```python
from build123d import *

# Parameters (mm, degrees)
V4_UPPER_DECK_221X142_PROFILE_W  = 221
V4_UPPER_DECK_221X142_PROFILE_H  = 142
V4_UPPER_DECK_5MM_DEPTH          = 5
V4_FIVE_SUPPORT_POSTS_PROFILE_W  = 16
V4_FIVE_SUPPORT_POSTS_PROFILE_H  = 16
V4_FIVE_SUPPORT_POSTS_59MM_DEPTH = 59
V4_UPPER_TWO_CABLE_SLOTS_DEPTH   = 5.5
V4_FIVE_M3_PILOTS_PROFILE_R      = 1.4
V4_POST_PILOT_HOLES_DEPTH        = 14


with BuildPart() as part:
    # V4_upper_deck_221x142_profile → V4_upper_deck_5mm (new body)
    with BuildSketch(Plane(origin=(0, 4, 0), x_dir=(1, 0, 0), z_dir=(0, 1, 0))):
        with Locations((12.5, -115)):
            Rectangle(V4_UPPER_DECK_221X142_PROFILE_W, V4_UPPER_DECK_221X142_PROFILE_H)
    extrude(amount=-V4_UPPER_DECK_5MM_DEPTH)

    # V4_five_support_posts_profile → V4_five_support_posts_59mm (add)
    with BuildSketch(Plane(origin=(0, -1, 0), x_dir=(1, 0, 0), z_dir=(0, 1, 0))):
        with Locations((-85, -60)):
            Rectangle(V4_FIVE_SUPPORT_POSTS_PROFILE_W, V4_FIVE_SUPPORT_POSTS_PROFILE_H)
        with Locations((110, -60)):
            Rectangle(V4_FIVE_SUPPORT_POSTS_PROFILE_W, V4_FIVE_SUPPORT_POSTS_PROFILE_H)
        with Locations((-85, -171)):
            Rectangle(V4_FIVE_SUPPORT_POSTS_PROFILE_W, V4_FIVE_SUPPORT_POSTS_PROFILE_H)
        with Locations((110, -171)):
            Rectangle(V4_FIVE_SUPPORT_POSTS_PROFILE_W, V4_FIVE_SUPPORT_POSTS_PROFILE_H)
        with Locations((12.5, -130)):
            Rectangle(V4_FIVE_SUPPORT_POSTS_PROFILE_W, V4_FIVE_SUPPORT_POSTS_PROFILE_H)
    extrude(amount=-V4_FIVE_SUPPORT_POSTS_59MM_DEPTH)

    # V4_upper_two_cable_slots_profile → V4_upper_two_cable_slots (cut)
    with BuildSketch(Plane(origin=(0, 4, 0), x_dir=(1, 0, 0), z_dir=(0, 1, 0))):
        with BuildLine():
            Line((-11, -51), (-5, -51))
            ThreePointArc((-5, -51), (-1, -55), (-5, -59))
            Line((-5, -59), (-11, -59))
            ThreePointArc((-11, -59), (-15, -55), (-11, -51))
        make_face()
        with BuildLine():
            Line((20, -51), (26, -51))
            ThreePointArc((26, -51), (30, -55), (26, -59))
            Line((26, -59), (20, -59))
            ThreePointArc((20, -59), (16, -55), (20, -51))
        make_face()
    extrude(amount=-V4_UPPER_TWO_CABLE_SLOTS_DEPTH, mode=Mode.SUBTRACT)

    # V4_five_M3_pilots_profile → V4_post_pilot_holes (cut)
    with BuildSketch(Plane(origin=(0, -60, 0), x_dir=(1, 0, 0), z_dir=(0, 1, 0))):
        with Locations(Location((-85, -60, 0), (0, 0, 270))):
            Circle(V4_FIVE_M3_PILOTS_PROFILE_R)
        with Locations(Location((110, -60, 0), (0, 0, 270))):
            Circle(V4_FIVE_M3_PILOTS_PROFILE_R)
        with Locations(Location((-85, -171, 0), (0, 0, 270))):
            Circle(V4_FIVE_M3_PILOTS_PROFILE_R)
        with Locations(Location((110, -171, 0), (0, 0, 270))):
            Circle(V4_FIVE_M3_PILOTS_PROFILE_R)
        with Locations(Location((12.5, -130, 0), (0, 0, 270))):
            Circle(V4_FIVE_M3_PILOTS_PROFILE_R)
    extrude(amount=V4_POST_PILOT_HOLES_DEPTH, mode=Mode.SUBTRACT)


solid = part.part
```
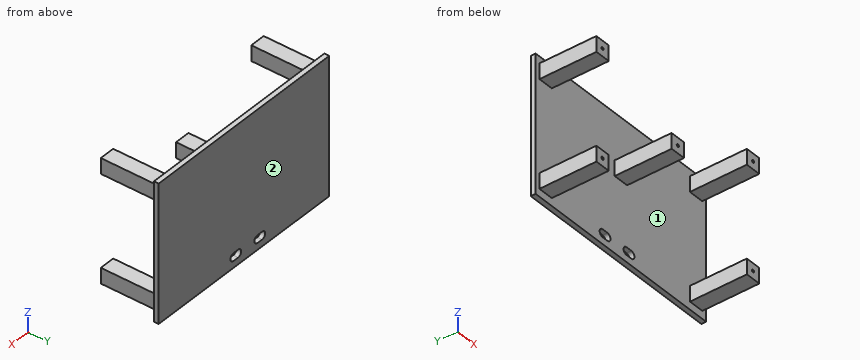
The listing builds one solid part. Answer for the finished solid, in the listing's coordinates (mm). Face numbers are marked on the shaded views. Coordinates: 2 decimals unless noted, no trailing zeros. Order: outer loops, then holes, each group sorted by start corner. A loop starts at its lowest first (then second) coordinate and runs counter-clockwise, first axis right, second up. Notation, with made-up numbers: M 6.5,25.25 L 42.5,25.25 A23 ccw 42.5,53.25 Z; hole C 17,24.5 d7. An arc over 180 degrees is marked long. Answer as a JSON object with one key per item and string values. Group by question number.
1. Flat-ended cylindrical pins translate along their axes: P1, Ø4, axis at x = -42, z = 153, coming from the -Y side; P2, Ø5, axis at y = -20, z = 62.5, coming from the -X side; P3, Ø2, axis at x = -84.5, z = 60.5, coming from the -Y side; P4, Ø8, axis at x = 107.5, y = -22, coming from the -Z side. Find the tip coordinate at first contact, or state that the pin passes through.
2. Straight lines are drawn through the part: line 1 (X direction, y = -51, z = 171); line 2 (Z direction, x = 110, y = -52); line 3 (X direction, y = -56.75, z = 130). For each, find the intervals that lie inside material, in ascending order.
3. Section C-C on z = 55 is taken. Write down the section's boundary in (x, y).
4. Determine the mould class of the marked faces 1 and 2 for opening direction X: released by +X, released by -X, zero draft, split by the parting line, or undercut.
5. Section B-B on y = -7 is taken. Write down the section's boundary in (x, z), then the cut area to 3 significant figures.
6. Section D-D on z = 176 is taken. Write down the section's boundary in (x, y).
7. Section A-A on y = -52 is taken. State how many separate pieces and enclosed holes the cut face has, then the cut area to 3 significant figures.
Values follow:
{
 "1": {"P1": "y = -1", "P2": "x = -93", "P3": "y = -60", "P4": "z = 52"},
 "2": {"line 1": "-93 to -86.4, -83.6 to -77, 102 to 108.6, 111.4 to 118", "line 2": "52 to 58.6, 61.4 to 68, 163 to 169.6, 172.4 to 179", "line 3": "4.5 to 11.1, 13.9 to 20.5"},
 "3": {"outline": "M -98,-1 L -93,-1 L -93,-60 L -77,-60 L -77,-1 L -15,-1 L -15,4 L -98,4 Z; M -1,-1 L 16,-1 L 16,4 L -1,4 Z; M 30,-1 L 102,-1 L 102,-60 L 118,-60 L 118,-1 L 123,-1 L 123,4 L 30,4 Z"},
 "4": {"face 1": "undercut", "face 2": "zero draft"},
 "5": {"outline": "M -93,52 L -77,52 L -77,68 L -93,68 Z; M -93,163 L -77,163 L -77,179 L -93,179 Z; M 4.5,122 L 20.5,122 L 20.5,138 L 4.5,138 Z; M 102,52 L 118,52 L 118,68 L 102,68 Z; M 102,163 L 118,163 L 118,179 L 102,179 Z", "area": "1,280 mm2"},
 "6": {"outline": "M -98,-1 L -93,-1 L -93,-60 L -77,-60 L -77,-1 L 102,-1 L 102,-60 L 118,-60 L 118,-1 L 123,-1 L 123,4 L -98,4 Z"},
 "7": {"separate pieces": "5", "enclosed holes": "5", "area": "1,250 mm2"}
}
